Job drawing, mm, ordinate dimensions from the low corner. One solid piece. A direction names the side the tool comes from. Coordinates: 2 decimals unless noted, no trailing zeros. Order: outer loops, then holes, each group sorted by start corner. A loop starts at its lowest first (then second) coordinate and runs counter-clockwise, first axis right, second up. Notation, with made-up numbers: (49.25, 68) - (90.25, 68) arc R12 ccw to (90.25, 75) - close; hole circle Ø2 at (-37.5, -27.75). An arc over 180 degrees is marked (long way). Use one line per item in the form item = value.
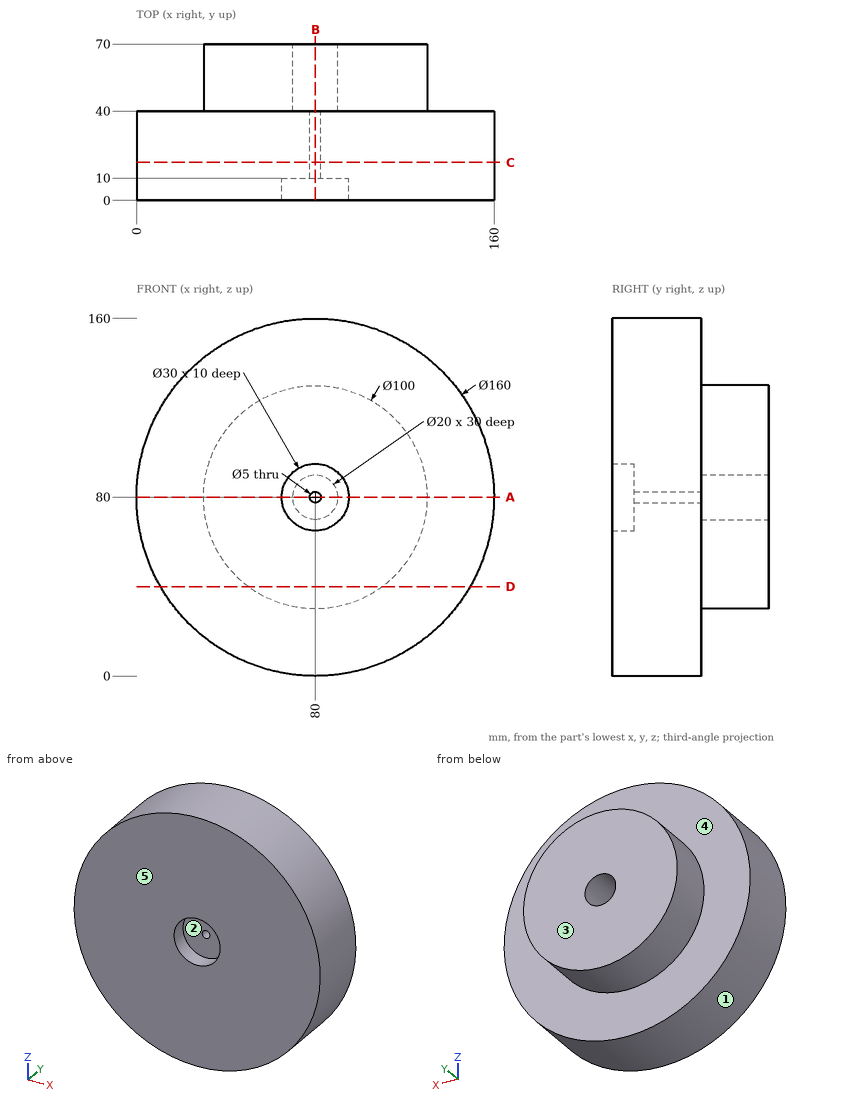
Item 1: Drop flat-ended pins along their axis: pin 1 (1 mm diameter, centred on y = 28.5, z = 51, fed in from +X); pin 2 (3 mm diameter, centred on y = 36, z = 140.5, fed in from -X); pin 3 (18 mm diameter, centred on x = 80, z = 80, fed in from +Y); pin 4 (4.5 mm diameter, centred on x = 80, z = 80, fed in from +Y). Give the stop position or say it passes through.
Derived:
pin_1 = 154.75
pin_2 = 25.97
pin_3 = 40
pin_4 = through
Item 2: 3-axis set-ups, long thin cutter, end or side, ignore diameter. For the marked faces 4 and 5: which of +Z, -Z, +X, -X, +Y, -Y reach the whole face in a straight line?
Derived:
face_4 = +Y
face_5 = +Z, -Z, +X, -X, -Y
Item 3: Cut at D-D, the plane z = 40. Write the cut outline in (x, y).
Derived:
outline = (10.72, 0) - (149.28, 0) - (149.28, 40) - (110, 40) - (110, 70) - (50, 70) - (50, 40) - (10.72, 40) - close
Item 4: Cut at C-C, the plane y = 17. Write the cut outline in (x, z), plus the area to 3 significant figures.
Derived:
outline = circle Ø160 at (80, 80); hole circle Ø5 at (80, 80)
area = 20,100 mm²
Item 5: Cut at B-B, the plane x = 80. Write the cut outline in (y, z), plus the area to 3 significant figures.
Derived:
outline = (0, 0) - (40, 0) - (40, 30) - (70, 30) - (70, 70) - (40, 70) - (40, 77.5) - (10, 77.5) - (10, 65) - (0, 65) - close; (0, 95) - (10, 95) - (10, 82.5) - (40, 82.5) - (40, 90) - (70, 90) - (70, 130) - (40, 130) - (40, 160) - (0, 160) - close
area = 8,350 mm²
Item 6: Drill centre lines: line 1 (X direction, y = 62.25, z = 80); line 2 (Y direction, x = 100.5, z = 141.5). Where is each one in solid material? Low to high. Write a range as [from, to].
Derived:
line_1 = [30, 70], [90, 130]
line_2 = [0, 40]
Item 7: Cut at A-A, the plane z = 80. Write the cut outline in (x, y).
Derived:
outline = (0, 0) - (65, 0) - (65, 10) - (77.5, 10) - (77.5, 40) - (70, 40) - (70, 70) - (30, 70) - (30, 40) - (0, 40) - close; (82.5, 10) - (95, 10) - (95, 0) - (160, 0) - (160, 40) - (130, 40) - (130, 70) - (90, 70) - (90, 40) - (82.5, 40) - close
Item 8: Two-plate mould, pull along X, no slides. Class the marked faces 1, 2 and 3: +X half, -X half, draft (parallel to the pull), parting line (faces both ways), or undercut.
Derived:
face_1 = parting line
face_2 = undercut
face_3 = draft
